Input: part model. Units: mm. Frame: model coordinates. A direction names the side the tool comes from. Round coordinates to 2 decimals unless told otherwise and drop trailing zeros. Loops run counter-clockwise (first coordinate to the right, second up) from the corner with the lowest first, then second, coordinate; pieces in that order, holes last. Notation, with made-up numbers: M -15.5,82.5 L -2.5,82.5 A25 ccw -2.5,113.5 Z; hole C 48.5,53.25 d5. An arc over 180 degrees is marked long. Return JSON: item names as keys, results as strings. Group by question number.
1) Contact query for flat-ended pins moving along their axis: P1, Ø4, axis at x = -49, y = 19.5, coming from the +Z side; P2, Ø2, axis at y = 22, z = 18.5, coming from the +X side; P3, Ø6, axis at x = -72.5, z = 16, coming from the +Y side. Output: stop coordinate, or through.
2) Section A-A (z = 46). Output: boundary loops of the cut face in (x, y).
3) Section B-B (z = 18). Output: boundary loops of the cut face in (x, y), plus the area to 3 significant figures.
4) Material intervals for line 1 (Z direction, x = -68.5, y = 14); line 2 (Y direction, x = -60, z = 4); line 3 (Y direction, x = -51, z = 8), sorted ascending. Write a range as from..to.
5) Access query for faces 1 (the face through (-58.102, 24.695, 45.005)), 2 (the face through (-77.05, 24.04, 18.8)). Directions: +Z, -Z, +X, -X, +Y, -Y. A direction counts if a zero-diameter tool reaches every point of the face in a straight line with its end or side. Return the directions, or none.
from build123d import *

# Parameters (mm, degrees)
F0_R     = 17.526
F1_DEPTH = 38.1
F2_R     = 1.9304
F3_DEPTH = 50.8
F4_R     = 1.27


with BuildPart() as f1:
    # F0 (on Top) → F1 (new body)
    with BuildSketch(Plane.XY):
        with Locations((-59.5418959856, 23.2741720974)):
            Circle(F0_R)
    extrude(amount=F1_DEPTH)

    # F2 (on Top) → F3 (join)
    with BuildSketch(Plane.XY):
        with Locations((-59.9432475865, 24.1154804826)):
            Circle(F2_R)
    extrude(amount=F3_DEPTH)

    # F4
    f4_edges = [f1.edges().sort_by_distance(p)[0] for p in [
        (-77.067896, 23.274172, 38.1),
        (-61.873648, 24.11548, 38.1),
        (-77.067896, 23.274172, 0),
    ]]
    fillet(f4_edges, radius=F4_R)


solid = f1.part
Returned:
{
 "1": {"P1": "stops at z = 38.1", "P2": "stops at x = -42.02", "P3": "stops at y = 37.7"},
 "2": {"outline": "C -59.94,24.12 d3.86"},
 "3": {"outline": "C -59.54,23.27 d35.05", "area": "965 mm^2"},
 "4": {"line 1": "z = 0..38.1", "line 2": "y = 5.75..40.79", "line 3": "y = 7.97..38.58"},
 "5": {"face 1": "+Z", "face 2": "+Z, -Z"}
}
